The model under review builds one solid part; all positions refer to its coordinate system, in mm. A direction names the side the tool comes from. Give positions to 0.01 mm unless a question says otherwise; leave off trailing zeros. Order: outer loops, then holes, each group sorted by start corner. A loop starts at its lowest first (then second) coordinate and runs counter-clockwise, first axis right, second up. Notation, with made-up numbers: (61.5, 55.25) - (100.5, 55.25) arc R10 ccw to (100.5, 67.25) - close; hole circle Ø9 at (-16, 65). An arc over 180 degrees is marked (long way). Use CSV: the item, a comma, the result in double quotes. Start each with the question number.
```python
from build123d import *

# Parameters (mm, degrees)
SKETCH2_R           = 20.5
BOSS_EXTRUDE1_DEPTH = 4
BOSS_EXTRUDE2_START = -2
BOSS_EXTRUDE2_DEPTH = 2
SKETCH4_R           = 0.75
SKETCH4_W           = 13
SKETCH4_H           = 24
BOSS_EXTRUDE3_DEPTH = 5
SKETCH5_W           = 10
SKETCH5_H           = 5
BOSS_EXTRUDE4_DEPTH = 25
SKETCH6_W           = 21
SKETCH6_H           = 7
BOSS_EXTRUDE5_DEPTH = 52.4
SKETCH7_R           = 1.6
CUT_EXTRUDE1_DEPTH  = 52.4
SKETCH8_R           = 0.500000007
CUT_EXTRUDE2_DEPTH  = 10
SKETCH9_W           = 8.5
SKETCH9_H           = 24
CUT_EXTRUDE3_DEPTH  = 10
SKETCH10_W          = 10
SKETCH10_H          = 2.505647768
BOSS_EXTRUDE6_DEPTH = 31
SKETCH11_W          = 10
SKETCH11_H          = 24.604481137
SKETCH11_R          = 1.7
BOSS_EXTRUDE7_DEPTH = 4
BOSS_EXTRUDE8_DEPTH = 5
SKETCH13_W          = 11.098107646
SKETCH13_H          = 34.722384721
CUT_EXTRUDE4_DEPTH  = 10


with BuildPart() as part:
    # Sketch2 → Boss-Extrude1 (new body)
    with BuildSketch(Plane.XY):
        with Locations((-30.000000447, 0)):
            Circle(SKETCH2_R)
        with BuildLine():
            Line((-32.000000447, -13.925), (-32.700000447, -2.147673159))
            ThreePointArc((-32.700000447, -2.147673159), (-33.450000447, 0), (-32.700000447, 2.147673159))
            Line((-32.700000447, 2.147673159), (-32.000000447, 13.925))
            ThreePointArc((-32.000000447, 13.925), (-30.000000447, 15.925), (-28.000000447, 13.925))
            Line((-28.000000447, 13.925), (-27.300000447, 2.147673159))
            ThreePointArc((-27.300000447, 2.147673159), (-26.550000447, 0), (-27.300000447, -2.147673159))
            Line((-27.300000447, -2.147673159), (-28.000000447, -13.925))
            ThreePointArc((-28.000000447, -13.925), (-30.000000447, -15.925), (-32.000000447, -13.925))
        make_face(mode=Mode.SUBTRACT)
    extrude(amount=-BOSS_EXTRUDE1_DEPTH)

    # Sketch3 → Boss-Extrude2 (add)
    with BuildSketch(Plane(origin=(0, 0, -4), x_dir=(-1, 0, 0), z_dir=(0, 0, -1)).offset(BOSS_EXTRUDE2_START)):
        with BuildLine():
            Line((32.000000447, 13.925), (32.700000447, 2.147673159))
            ThreePointArc((32.700000447, 2.147673159), (30.000000278, 3.45000035), (27.300000447, 2.147673159))
            Line((27.300000447, 2.147673159), (28.000000447, 13.925))
            ThreePointArc((28.000000447, 13.925), (30.000000447, 15.925), (32.000000447, 13.925))
        make_face()
        with BuildLine():
            Line((32.700000447, -2.147673159), (32.000000447, -13.925))
            ThreePointArc((32.000000447, -13.925), (30.000000447, -15.925), (28.000000447, -13.925))
            Line((28.000000447, -13.925), (27.300000447, -2.147673159))
            ThreePointArc((27.300000447, -2.147673159), (30.000000278, -3.44999965), (32.700000447, -2.147673159))
        make_face()
    extrude(amount=BOSS_EXTRUDE2_DEPTH)

    # Sketch4 → Boss-Extrude3 (add)
    with BuildSketch(Plane.XY):
        Polygon((-45.000000447, 0), (-35.000000447, 0), (-35.000000447, 63.556554203), (-25.000000447, 63.556554203), (-25.000000447, 0), (-15.000000447, 0), (-15.000000447, 66.480727098), (-15.000000447, 108.20577925), (-45.000000447, 108.20577925), (-45.000000447, 66.480727098), align=None)
        with Locations((-30.000000447, 70.680727098)):
            Circle(SKETCH4_R, mode=Mode.SUBTRACT)
        with Locations((-30.000000447, 98.480727098)):
            Circle(SKETCH4_R, mode=Mode.SUBTRACT)
        with Locations((-30.000000447, 85.330727098)):
            Rectangle(SKETCH4_W, SKETCH4_H, mode=Mode.SUBTRACT)
    extrude(amount=BOSS_EXTRUDE3_DEPTH)

    # Sketch5 → Boss-Extrude4 (add)
    with BuildSketch(Plane(origin=(0, 0, 0), x_dir=(-1, 0, 0), z_dir=(0, 0, -1))):
        with Locations((40.000000447, 45.531062225)):
            Rectangle(SKETCH5_W, SKETCH5_H)
    extrude(amount=BOSS_EXTRUDE4_DEPTH)

    # Sketch6 → Boss-Extrude5 (add)
    with BuildSketch(Plane(origin=(0, 48.031062225, 0), x_dir=(1, 0, 0), z_dir=(0, 1, 0))):
        with Locations((-34.401892801, 21.5)):
            Rectangle(SKETCH6_W, SKETCH6_H)
    extrude(amount=BOSS_EXTRUDE5_DEPTH)

    # Sketch7 → Cut-Extrude1 (cut)
    with BuildSketch(Plane(origin=(0, 0, -25), x_dir=(-1, 0, 0), z_dir=(0, 0, -1))):
        with Locations((30.000000447, 89.730727098)):
            Circle(SKETCH7_R)
    extrude(amount=-CUT_EXTRUDE1_DEPTH, mode=Mode.SUBTRACT)

    # Sketch8 → Cut-Extrude2 (cut)
    with BuildSketch(Plane.XY):
        with Locations((-29.975317233, 10.434970799)):
            Circle(SKETCH8_R)
        with Locations((-30.020023773, -8.464976311)):
            Circle(SKETCH8_R)
    extrude(amount=-CUT_EXTRUDE2_DEPTH, mode=Mode.SUBTRACT)

    # Sketch9 → Cut-Extrude3 (cut)
    with BuildSketch(Plane.XY.offset(5)):
        with Locations((-19.250000447, 85.330727098)):
            Rectangle(SKETCH9_W, SKETCH9_H)
    extrude(amount=-CUT_EXTRUDE3_DEPTH, mode=Mode.SUBTRACT)

    # Sketch10 → Boss-Extrude6 (add)
    with BuildSketch(Plane.XY):
        with Locations((-30.000000447, 18.464419485)):
            Rectangle(SKETCH10_W, SKETCH10_H)
    extrude(amount=BOSS_EXTRUDE6_DEPTH)

    # Sketch11 → Boss-Extrude7 (add)
    with BuildSketch(Plane.XY.offset(31)):
        with Locations((-30.000000447, 7.415002801)):
            Rectangle(SKETCH11_W, SKETCH11_H)
        with Locations((-30.000000447, 0)):
            Circle(SKETCH11_R, mode=Mode.SUBTRACT)
    extrude(amount=-BOSS_EXTRUDE7_DEPTH)

    # Sketch12 → Boss-Extrude8 (add)
    with BuildSketch(Plane.XY.offset(5)):
        with BuildLine():
            Line((-14.181307682, 48.701973767), (-13.362614918, 51.064121552))
            ThreePointArc((-13.362614918, 51.064121552), (-10.487154092, 48.492549322), (-10.297966628, 44.639567777))
            Line((-10.297966628, 44.639567777), (-15.000000447, 31.636176901))
            Line((-15.000000447, 31.636176901), (-15.000000447, 43.839825982))
            ThreePointArc((-15.000000447, 43.839825982), (-12.534704373, 45.924717238), (-14.181307682, 48.701973767))
        make_face()
        with BuildLine():
            Line((-49.702034266, 44.639567777), (-45.000000447, 31.636176901))
            Line((-45.000000447, 31.636176901), (-45.000000447, 43.839825982))
            ThreePointArc((-45.000000447, 43.839825982), (-47.465296521, 45.924717238), (-45.818693212, 48.701973767))
            Line((-45.818693212, 48.701973767), (-46.637385976, 51.064121552))
            ThreePointArc((-46.637385976, 51.064121552), (-49.512846802, 48.492549322), (-49.702034266, 44.639567777))
        make_face()
    extrude(amount=-BOSS_EXTRUDE8_DEPTH)

    # Sketch13 → Cut-Extrude4 (cut)
    with BuildSketch(Plane(origin=(0, 0, -25), x_dir=(-1, 0, 0), z_dir=(0, 0, -1))):
        with Locations((29.450946624, 65.392254586)):
            Rectangle(SKETCH13_W, SKETCH13_H)
    extrude(amount=-CUT_EXTRUDE4_DEPTH, mode=Mode.SUBTRACT)


solid = part.part
```
1. Mouldability with a two-part tool opening along Z and no side actions: class faces 6 (the face through (-15, 103, 2)), 7 (the face through (-37, 80, -18)), 8 (the face through (-39, 55, 5)), 9 (the face through (-26, 0, -4)) as pulls with the +Z half, pulls with the -Z half, needs draft (parallel to the pull), parting line crosses it, or undercut.
2. Consider section B-B (x = -22). Give the boundary of the cut face in (y, z).
3. Consider section D-D (z = -10). Give the boundary of the cut face in (x, y), and give its area (3 significant figures).
4. Consider section C-C (x = -40.5). Give the boundary of the cut face in (y, z), and give its area (3 significant figures).
5. Clearance check with flat-ended pins moving along their axes: pin 1 (2.5 mm diameter, centred on y = 9, z = 2.5, fed in from +X); pin 2 (11 mm diameter, centred on x = -30, z = 14.5, fed in from +Y); pin 3 (2 mm diameter, centred on y = 42, z = -3.5, fed in from -X); pin 4 (8 mm diameter, centred on y = -5, z = -3.5, fed in from +X). State where each tip first meets the part, or that it passes through.
6. To check wall thickness, follow L1, parallel to Z at x = -40.5, y = 49; L2, parallel to Z at x = -27, y = 13.5; L3, parallel to Y at x = -30, z = -22. State the ranges of each line that lie inside material, in increasing order. Write a range as [from, to].
7. Consider section A-A (y = 22). Give the boundary of the cut face in (x, z).
8. Tool access review of faces 1 (the face through (-45, 16, 2)), 2 (the face through (-15, 58, 2)), 3 (the face through (-29, 82.753, -22)), 4 (the face through (-44.902, 74, -21)), 5 (the face through (-35, 12, 29)): name each direction out of +Z, -Z, +X, -X, +Y, -Y from which nothing blocks a thin tool from reaching the whole face with its end or side.
Answers follow:
1,face 6,"needs draft"
1,face 7,"undercut"
1,face 8,"pulls with the +Z half"
1,face 9,"pulls with the -Z half"
2,outline,"(-18.87, -4) - (18.87, -4) - (18.87, 0) - (73.33, 0) - (73.33, 5) - (0, 5) - (0, 0) - (-18.87, 0) - close; (97.33, 0) - (108.21, 0) - (108.21, 5) - (97.33, 5) - close"
3,outline,"(-45, 43.03) - (-35, 43.03) - (-35, 48.03) - (-45, 48.03) - close"
3,area,"50.0 mm^2"
4,outline,"(-17.61, -4) - (17.61, -4) - (17.61, 0) - (43.03, 0) - (43.03, -25) - (100.43, -25) - (100.43, -18) - (48.03, -18) - (48.03, 0) - (108.21, 0) - (108.21, 5) - (0, 5) - (0, 0) - (-17.61, 0) - close"
4,area,"1,170 mm^2"
5,pin 1,"stops at x = -15"
5,pin 2,"stops at y = 19.72"
5,pin 3,"passes through"
5,pin 4,"stops at x = -9.52"
6,L1,"z = [-25, -18], [0, 5]"
6,L2,"z = [-4, 0], [27, 31]"
6,L3,"y = [82.75, 88.13], [91.33, 100.43]"
7,outline,"(-45, 0) - (-35, 0) - (-35, 5) - (-45, 5) - close; (-25, 0) - (-15, 0) - (-15, 5) - (-25, 5) - close"
8,face 1,"+Z, -X, -Y"
8,face 2,"+Z, -Z, +Y"
8,face 3,"+Z, -Z, +X, -Y"
8,face 4,"-Z, -X, +Y"
8,face 5,"+Z, -X, +Y, -Y"
